Check sheet for the modelled part. Datum: model origin and axes. Units: mm. A direction names the side the tool comes from. Coordinates: 2 decimals unless noted, no trailing zeros. Write each loop counter-clockwise with the first axis right and the second up, starting at its lowest first coordinate (ties: lowest second). Pieces come first, ordered by that corner, then holes. Notation, with made-up numbers: M 45.5,8.25 L 78.5,8.25 A22 ccw 78.5,29.25 Z; hole C 41,31 d11. An arc over 180 degrees is marked long. Answer as CSV lines item,"result". Start each with the question number.
Q1. Thickness scan on line 1 along Z through (x, y) = (12.25, -5.5); line 2 along X through (y, z) = (20, 6); line 3 along X through (y, z) = (0, -11). Record the ranges inside material, lowest first. Write a range as from..to.
Q2. Sectioned sample at D-D, the plane z = 29. Record the cut outline in (x, y).
Q3. Sectioned sample at C-C, the plane y = 0. Record the cut outline in (x, z), then the cut area to 3 significant figures.
Q4. Sectioned sample at A-A, the plane z = 0. Record the cut outline in (x, y).
Q5. Depth check by flat-ended pin: pin 1 Ø8 at (y, z) = (0.5, -14) entering from +X; pin 2 Ø3.5 at (x, y) = (5.5, 33) entering from +Z; pin 3 Ø4 at (x, z) = (4, 21) entering from -Y. Enter the tip coordinate at first touch or a pass-through.
Q6. Access from +Z, -Z, +X, -X, +Y, -Y to the whole of each face (thin tool, end or side, straight path). Record for faces 1 (the flat face through (7, 0, -6)), 2 (the flat face through (7.6, -9.97, 32.27)), 3 (the cylindrical face through (8.958, -7.509, 23.846)).
Q7. Mould release check, pull along Z, two halves, no side actions. Record for faces 4 (the cylindrical face through (7.6, 0.1, 31.5)), 5 (the flat face through (7.6, -22.96, -24.77)), 6 (the flat face through (13, 0, 7)), 7 (the flat face through (0, 15.5, 0.5)): pulls with the +Z half, pulls with the -Z half, needs draft (parallel to the pull), parting line crosses it, or undercut.
Q8. Sectioned sample at B-B, the plane x = 3. Record the cut outline in (y, z), then the cut area to 3 significant figures.
from build123d import *

# Parameters (mm, degrees)
SKETCH_2_W               = 12
SKETCH_2_H               = 12
CUT_EXTRUDE_1_DEPTH      = 47.405818601
EXTRUDE_START            = -15
EXTRUDE_1_DEPTH          = 15
PATTERN_CIRCULAR_1_COUNT = 6
FILLET_1_R               = 2


with BuildPart() as part:
    # Эскиз1 → Повернуть1 (revolve)
    with BuildSketch(Plane.XY, mode=Mode.PRIVATE) as revolve_1_sk:
        with BuildLine():
            Line((2, 0), (2, 15))
            Line((2, 15), (0, 15))
            Line((0, 15), (0, 31.5))
            Line((0, 31.5), (15, 31.5))
            Line((15, 31.5), (15, 28))
            ThreePointArc((15, 28), (14.121320344, 25.878679656), (12, 25))
            Line((12, 25), (4, 25))
            Line((4, 25), (4, 17))
            Line((4, 17), (13, 17))
            Line((13, 17), (13, 0))
            Line((13, 0), (2, 0))
        make_face()
    revolve(revolve_1_sk.sketch.rotate(Axis((0, 0, 0), (1, 0, 0)), 90), axis=Axis((0, 0, 0), (1, 0, 0)))

    # Эскиз2 → Вырез-Вытянуть1 (cut, through all)
    with BuildSketch(Plane.ZY.offset(-2)):
        Rectangle(SKETCH_2_W, SKETCH_2_H)
    extrude(amount=-CUT_EXTRUDE_1_DEPTH, mode=Mode.SUBTRACT)

    # Эскиз3 → Бобышка-Вытянуть1 (add)
    with BuildSketch(Plane.ZY.offset(EXTRUDE_START)):
        with BuildLine():
            ThreePointArc((7.5, 35.210083783), (0, 36), (-7.5, 35.210083783))
            Line((-7.5, 35.210083783), (-7.5, 30.594117082))
            ThreePointArc((-7.5, 30.594117082), (0, 31.5), (7.5, 30.594117082))
            Line((7.5, 30.594117082), (7.5, 35.210083783))
        make_face()
    extrude_1 = extrude(amount=EXTRUDE_1_DEPTH)

    # Круговой массив1: Бобышка-Вытянуть1 ×6 about axis
    pattern_circular_1_axis = Axis((0, 0, 0), (1, 0, 0))
    for i in range(1, PATTERN_CIRCULAR_1_COUNT):
        add(extrude_1.rotate(pattern_circular_1_axis, i * 360 / PATTERN_CIRCULAR_1_COUNT))

    # Скругление1
    fillet_1_edges = [part.edges().sort_by_distance(p)[0] for p in [
        (4, 0, -17),
        (4, 0, -25),
    ]]
    fillet(fillet_1_edges, radius=FILLET_1_R)


solid = part.part
Output:
1,line 1,"z = -31.02..-24.4, -16.09..-6, 6..16.09, 24.4..31.02"
1,line 2,"x = 0..4"
1,line 3,"x = 2..13"
2,outline,"M 0,-21.33 L 15,-21.33 L 15,21.33 L 0,21.33 Z"
3,outline,"M 0,-31.5 L 15,-31.5 L 15,-28 A3 ccw 12,-25 L 6,-25 A2 cw 4,-23 L 4,-19 A2 cw 6,-17 L 13,-17 L 13,-6 L 2,-6 L 2,-15 L 0,-15 Z; M 0,15 L 2,15 L 2,6 L 13,6 L 13,17 L 6,17 A2 cw 4,19 L 4,23 A2 cw 6,25 L 12,25 A3 ccw 15,28 L 15,31.5 L 0,31.5 Z"
3,area,"509 mm^2"
4,outline,"M 0,-36 L 15,-36 L 15,-28 A3 ccw 12,-25 L 6,-25 A2 cw 4,-23 L 4,-19 A2 cw 6,-17 L 13,-17 L 13,-6 L 2,-6 L 2,-15 L 0,-15 Z; M 0,15 L 2,15 L 2,6 L 13,6 L 13,17 L 6,17 A2 cw 4,19 L 4,23 A2 cw 6,25 L 12,25 A3 ccw 15,28 L 15,36 L 0,36 Z"
5,pin 1,"stops at x = 13"
5,pin 2,"stops at z = 7.5"
5,pin 3,"stops at y = -25.12"
6,face 1,"+X, -X"
6,face 2,"+Z, +X, -X"
6,face 3,"+X"
7,face 4,"pulls with the +Z half"
7,face 5,"undercut"
7,face 6,"undercut"
7,face 7,"needs draft"
8,outline,"M -35.21,-7.5 L -30.59,-7.5 A31.5 ccw -21.79,-22.75 L -24.1,-26.74 A36 ccw -11.11,-34.24 L -8.8,-30.25 A31.5 ccw 8.8,-30.25 L 11.11,-34.24 A36 ccw 24.1,-26.74 L 21.79,-22.75 A31.5 ccw 30.59,-7.5 L 35.21,-7.5 A36 ccw 35.21,7.5 L 30.59,7.5 A31.5 ccw 21.79,22.75 L 24.1,26.74 A36 ccw 11.11,34.24 L 8.8,30.25 A31.5 ccw -8.8,30.25 L -11.11,34.24 A36 ccw -24.1,26.74 L -21.79,22.75 A31.5 ccw -30.59,7.5 L -35.21,7.5 A36 ccw Z; hole M -6,-6 L 6,-6 L 6,6 L -6,6 Z"
8,area,"3,380 mm^2"
